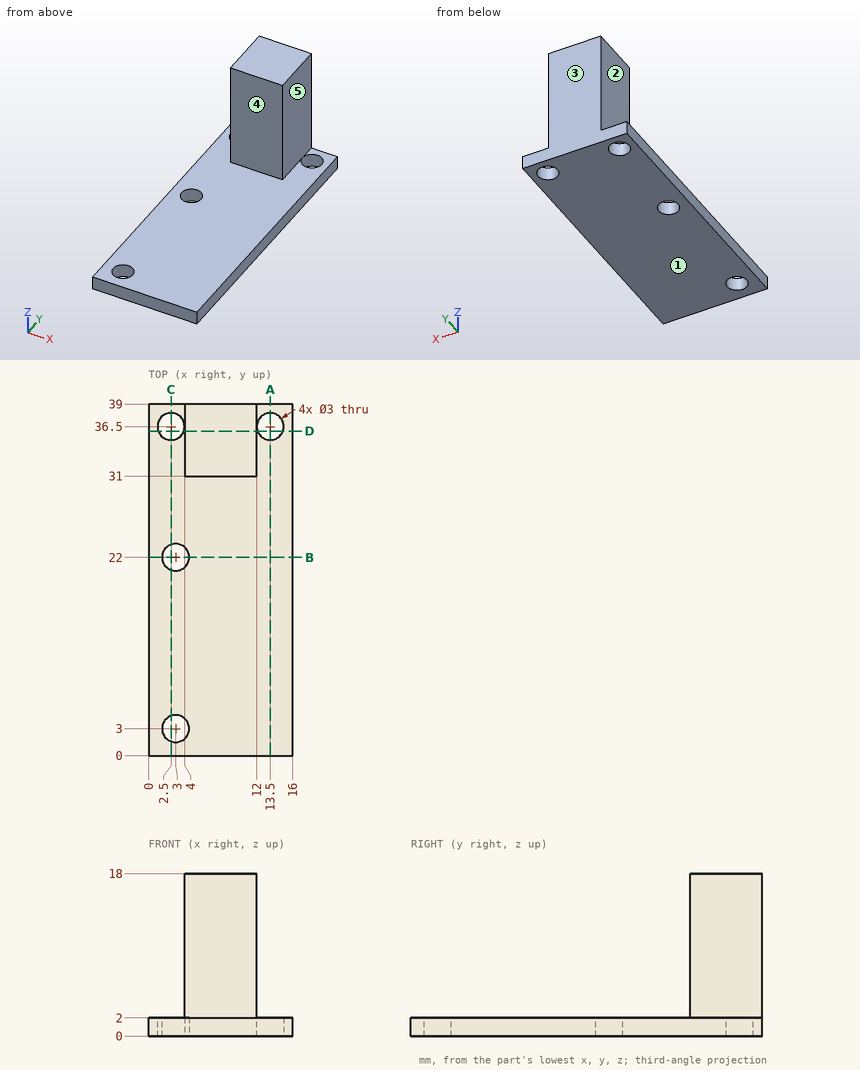
Geometry: see drawing. Coordinates: mm, zero at the bounding-box minimum. A direction names the side the tool comes from. Round coordinates to 2 decimals unless told otherwise and drop trailing zeros. Loops run counter-clockwise (first coordinate to the right, second up) from the corner with the lowest first, then second, coordinate; pieces in that order, holes last. Notation, with made-up numbers: (29.5, 46.25) - (82.5, 46.25) arc R11 ccw to (82.5, 51.25) - close; hole circle Ø8 at (1.5, 49). An arc over 180 degrees is marked (long way). Write item = value, one per line. Start each with the question number.
(1) Pin query (flat end, axial travel): pin 1 (2.5 mm diameter, centred on x = 2.5, y = 36.5, fed in from -Z); pin 2 (8 mm diameter, centred on x = 6, y = 13, fed in from +Z); pin 3 (3 mm diameter, centred on x = 5, z = 6, fed in from -Y); pin 4 (4 mm diameter, centred on y = 33.5, z = 12.5, fed in from +X). Return the tip coordinate at first contact, or that it passes through.
(2) Section query C-C, the plane x = 2.5. Output: boundary loops of the cut face in (y, z), plus the area to 3 significant figures.
(3) Pull-direction query (Y, two-part tool) for the marked faces 3, 4 and 5; classes: +Y half, -Y half, draft (parallel to the pull), parting line (faces both ways), or undercut.
(4) Section query A-A, the plane x = 13.5. Output: boundary loops of the cut face in (y, z).
(5) Section query B-B, the plane y = 22. Output: boundary loops of the cut face in (x, z), plus the area to 3 significant figures.
(6) Ray query, line 1 along Y through (x, z) = (13.5, 0.8); line 2 along Y through (x, z) = (2.5, 1); line 3 along Y through (x, z) = (6.75, 4). Return the intervals inside material, ascending. Write a range as from..to.
(7) Set-up query: the marked faces 1 and 2. Return all of +Z, -Z, +X, -X, +Y, -Y with unobstructed straight access to the full face (end or side cutting, diameter ignored); none if empty.
(8) Section query D-D, the plane y = 36. Output: boundary loops of the cut face in (x, z).
Conclusion:
q1.pin_1 = through
q1.pin_2 = 2
q1.pin_3 = 31
q1.pin_4 = 12
q2.outline = (0, 0) - (1.59, 0) - (1.59, 2) - (0, 2) - close; (4.41, 0) - (20.59, 0) - (20.59, 2) - (4.41, 2) - close; (23.41, 0) - (35, 0) - (35, 2) - (23.41, 2) - close; (38, 0) - (39, 0) - (39, 2) - (38, 2) - close
q2.area = 60.7 mm2
q3.face_3 = +Y half
q3.face_4 = -Y half
q3.face_5 = draft
q4.outline = (0, 0) - (35, 0) - (35, 2) - (0, 2) - close; (38, 0) - (39, 0) - (39, 2) - (38, 2) - close
q5.outline = (0, 0) - (1.5, 0) - (1.5, 2) - (0, 2) - close; (4.5, 0) - (16, 0) - (16, 2) - (4.5, 2) - close
q5.area = 26.0 mm2
q6.line_1 = 0..35, 38..39
q6.line_2 = 0..1.59, 4.41..20.59, 23.41..35, 38..39
q6.line_3 = 31..39
q7.face_1 = -Z, +X, -X, +Y, -Y
q7.face_2 = +Z, -X, +Y, -Y
q8.outline = (0, 0) - (1.09, 0) - (1.09, 2) - (0, 2) - close; (3.91, 0) - (12.09, 0) - (12.09, 2) - (12, 2) - (12, 18) - (4, 18) - (4, 2) - (3.91, 2) - close; (14.91, 0) - (16, 0) - (16, 2) - (14.91, 2) - close
